Check sheet for the modelled part. Datum: model origin and axes. Units: mm. A direction names the side the tool comes from. Give positions to 0.01 mm unless a question says otherwise; leave off trailing zeros. Loops run counter-clockwise (first coordinate to the right, second up) from the corner with the lowest first, then second, coordinate; pieces in that order, holes last.
```python
from build123d import *

# Parameters (mm, degrees)
BOSS_EXTRUDE1_DEPTH = 6.35
SKETCH3_W           = 16.2814
SKETCH3_H           = 177.8
BOSS_EXTRUDE2_DEPTH = 38.1
SKETCH5_R           = 6.75767
CUT_EXTRUDE1_DEPTH  = 194.57627713
SKETCH6_R           = 8.7641176
CUT_EXTRUDE2_DEPTH  = 11.3284
FILLET1_R           = 3.175


with BuildPart() as part:
    # Sketch1 → Boss-Extrude1 (new, symmetric)
    with BuildSketch(Plane.XY):
        with BuildLine():
            Line((110.652882407, 187.698930688), (94.371482407, 187.698930688))
            Line((94.371482407, 187.698930688), (94.371482407, 174.998930688))
            ThreePointArc((94.371482407, 174.998930688), (98.86911538, 171.662815624), (100.714782785, 166.375862067))
            Line((100.714782785, 166.375862067), (102.511582984, 118.494891962))
            Line((102.511582984, 118.494891962), (105.473932974, 39.554455817))
            ThreePointArc((105.473932974, 39.554455817), (102.530659302, 30.319876353), (94.371482407, 25.088418602))
            Line((94.371482407, 25.088418602), (94.371482407, 9.898930688))
            Line((94.371482407, 9.898930688), (110.652882407, 9.898930688))
            Line((110.652882407, 9.898930688), (110.652882407, 187.698930688))
        make_face()
    extrude(amount=BOSS_EXTRUDE1_DEPTH, both=True)

    # Sketch3 → Boss-Extrude2 (add)
    with BuildSketch(Plane(origin=(0, 0, -6.35), x_dir=(-1, 0, 0), z_dir=(0, 0, -1))):
        with Locations((-102.512182407, 98.798930688)):
            Rectangle(SKETCH3_W, SKETCH3_H)
    extrude(amount=BOSS_EXTRUDE2_DEPTH)

    # Sketch5 → Cut-Extrude1 (cut, through all)
    with BuildSketch(Plane.ZY.offset(-94.371482407)):
        with Locations(Location((-20.574, 148.010668688, 0), (0, 0, 270))):
            Circle(SKETCH5_R)
        with Locations(Location((-20.574, 49.587192688, 0), (0, 0, 270))):
            Circle(SKETCH5_R)
    extrude(amount=-CUT_EXTRUDE1_DEPTH, mode=Mode.SUBTRACT)

    # Sketch6 → Cut-Extrude2 (cut)
    with BuildSketch(Plane.ZY.offset(-94.371482407)):
        with Locations(Location((-20.574, 148.010668688, 0), (0, 0, 270))):
            Circle(SKETCH6_R)
        with Locations(Location((-20.574, 49.587192688, 0), (0, 0, 270))):
            Circle(SKETCH6_R)
    extrude(amount=-CUT_EXTRUDE2_DEPTH, mode=Mode.SUBTRACT)

    # Fillet1
    fillet1_edges = [part.edges().sort_by_distance(p)[0] for p in [
        (94.371482407, 25.088418602, 0),
        (94.371482407, 174.998930688, 0),
    ]]
    fillet(fillet1_edges, radius=FILLET1_R)


solid = part.part
```
(1) Section check C-C on y = 85. Record the boundary of the cut face in (x, z), plus the area to 3 significant figures.
(2) Section check B-B on z = -18.5. Record the boundary of the cut face in (x, y), plus the area to 3 significant figures.
(3) Section check D-D on y = 117. Record the boundary of the cut face in (x, z), plus the area to 3 significant figures.
(4) Gauge pin test, flat ends, axial feed: pin 1 Ø5.5 at (y, z) = (47, -17) entering from -X; pin 2 Ø3 at (y, z) = (117.5, -0.5) entering from -X; pin 3 Ø5.5 at (x, y) = (97.5, 62.5) entering from +Z. Record the tip position at first contact, or that the pin passes through.
(5) Access from +Z, -Z, +X, -X, +Y, -Y to the whole of each face (thin tool, end or side, straight path). Record for faces 5 (the face through (99.32, 170.99, 0.09)), 6 (the face through (103, 187.699, -19)), 7 (the face through (105.7, 45, -26)).
(6) Release check for a two-part mould opening along Z. For faces 1 (the face through (108.142, 141.565, -18.544)), 2 (the face through (94.91, 24.52, 0.09)), 3 (the face through (103, 100, -44.45)), 4 (the face through (99, 101, -6.35)) record: pulls with the +Z half, pulls with the -Z half, needs draft (parallel to the pull), parting line crosses it, or undercut.
(7) Section check A-A on y = 144. Record the boundary of the cut face in (x, z), plus the area to 3 significant figures.
(8) Material ranges on line 1 (Y direction, x = 102.25, z = -25.5); line 2 (Y direction, x = 104, z = -24.5); line 3 (Z direction, x = 101.5, y = 33), recorded low to high.
Computed values:
1. outline: (94.37, -44.45) - (110.65, -44.45) - (110.65, 6.35) - (103.77, 6.35) - (103.77, -6.35) - (94.37, -6.35) - close
1. area: 708 mm2
2. outline: (94.37, 9.9) - (110.65, 9.9) - (110.65, 43.16) - (105.7, 43.16) - (105.7, 41.07) - (94.37, 41.07) - close; (94.37, 58.1) - (105.7, 58.1) - (105.7, 56.02) - (110.65, 56.02) - (110.65, 141.58) - (105.7, 141.58) - (105.7, 139.5) - (94.37, 139.5) - close; (94.37, 156.53) - (105.7, 156.53) - (105.7, 154.44) - (110.65, 154.44) - (110.65, 187.7) - (94.37, 187.7) - close
2. area: 2,380 mm2
3. outline: (94.37, -44.45) - (110.65, -44.45) - (110.65, 6.35) - (102.57, 6.35) - (102.57, -6.35) - (94.37, -6.35) - close
3. area: 723 mm2
4. pin 1: stops at x = 105.7
4. pin 2: stops at x = 102.49
4. pin 3: stops at z = -6.35
5. face 5: +Z, -X
5. face 6: +Z, -Z, +X, -X, +Y
5. face 7: -X
6. face 1: undercut
6. face 2: needs draft
6. face 3: pulls with the -Z half
6. face 4: pulls with the +Z half
7. outline: (94.37, -44.45) - (110.65, -44.45) - (110.65, -26.01) - (105.7, -26.01) - (105.7, -28.37) - (94.37, -28.37) - close; (94.37, -12.78) - (105.7, -12.78) - (105.7, -15.14) - (110.65, -15.14) - (110.65, 6.35) - (101.55, 6.35) - (101.55, -6.35) - (94.37, -6.35) - close
7. area: 505 mm2
8. line 1: y = 9.9 to 42.34, 56.84 to 140.76, 155.26 to 187.7
8. line 2: y = 9.9 to 41.75, 57.42 to 140.18, 155.85 to 187.7
8. line 3: z = -44.45 to -6.35
